Autodesk Inventor part; units mm, degrees
ref_plane "YZ Plane" through (0, 0, 0) normal (1, 0, 0) x (0, 1, 0)
ref_plane "XZ Plane" through (0, 0, 0) normal (0, 1, 0) x (-1, 0, 0)
ref_plane "XY Plane" through (0, 0, 0) normal (0, 0, 1) x (1, 0, 0)
sketch "Sketch1" plane through (0, 0, 0) normal (0, 0, 1) x (1, 0, 0)
  line L0 (17.9921, 17.8802) -> (17.9921, -20.5689)
  line L1 (-32.0079, 4.8802) -> (-32.0079, 14.8802) construction
  line L2 (-32.0079, 14.8802) -> (-22.0079, 14.8802) construction
  line L3 (-22.0079, 14.8802) -> (-22.0079, 4.8802) construction
  line L4 (-22.0079, 4.8802) -> (-32.0079, 4.8802) construction
  line L5 (-32.0079, 4.8802) -> (-32.0079, 14.8802) construction
  line L6 (17.9921, 14.8802) -> (-31.6168, 14.8802) construction
  line L7 (-31.6168, 4.8802) -> (18.3832, 4.8802) construction
  line L8 (-22.0079, 14.8802) -> (17.9921, 14.8802)
  line L9 (17.9921, 11.8802) -> (-22.0079, 11.8802)
  line L10 (-22.0079, 11.8802) -> (-22.0079, 14.8802)
  line L11 (17.9921, 14.8802) -> (17.9921, 11.8802)
  line L12 (-25.0079, 14.8802) -> (17.9921, 14.8802)
  line L13 (17.9921, 14.8802) -> (17.9921, 17.8802)
  line L14 (17.9921, 17.8802) -> (-25.0079, 17.8802)
  line L15 (-25.0079, 17.8802) -> (-25.0079, 14.8802)
  point P0 (0, 0)
  dimension "d2" = 10
  dimension "d13" = 10
  dimension "d52" = 3
  dimension "d53" = 0
  dimension "d55" = 80
  dimension "d56" = 40
  dimension "d57" = 3
  dimension "d58" = 3
revolve "Revolution1" add sketch "Sketch1" angle 360 about axis through (17.9921, 17.8802, 0) along (0, -1, 0)
sketch "Sketch3" plane through (17.9921, 11.8802, 0) normal (0, -1, 0) x (1, 0, 0)
  circle A0 centre (0, 0) radius 40
  line L0 (0, 40) -> (0, -38.6275)
  line L1 (-39.9999, 0.0946) -> (39.9999, 0.0946)
  circle A1 centre (10, 0.0946) radius 2
  circle A2 centre (20, 0.0946) radius 2
  circle A3 centre (30, 0.0946) radius 2
  circle A4 centre (4.9181, 8.7075) radius 2
  circle A5 centre (9.9181, 17.3678) radius 2
  circle A6 centre (14.9181, 26.028) radius 2
  circle A7 centre (-5.0819, 8.613) radius 2
  circle A8 centre (-10.0819, 17.2732) radius 2
  circle A9 centre (-15.0819, 25.9335) radius 2
  circle A10 centre (-10, -0.0946) radius 2
  circle A11 centre (-20, -0.0946) radius 2
  circle A12 centre (-30, -0.0946) radius 2
  circle A13 centre (-4.9181, -8.7075) radius 2
  circle A14 centre (-9.9181, -17.3678) radius 2
  circle A15 centre (-14.9181, -26.028) radius 2
  circle A16 centre (5.0819, -8.613) radius 2
  circle A17 centre (10.0819, -17.2732) radius 2
  circle A18 centre (15.0819, -25.9335) radius 2
  circle A19 centre (0, 35.25) radius 1.75
  circle A20 centre (-30.5274, -17.625) radius 1.75
  circle A21 centre (30.5274, -17.625) radius 1.75
  circle A22 centre (0, 0) radius 37 construction
  point P0 (-17.9921, 0)
  dimension "d59" = 4
  dimension "d60" = 10
  dimension "d66" = 10
  dimension "d70" = 360
  dimension "d72" = 3.5
  dimension "d75" = 360
  dimension "d80" = 3
extrude "Extrusion2" cut sketch "Sketch3" against normal through all contours A3 L1 | L1 A3 | A12 L1 | L1 A12 | A19 L0 | L0 A19 | A2 L1 | L1 A2 | A11 L1 | L1 A11 | A10 L1 | L1 A10 | A1 L1 | L1 A1 | A4 | A5 | A6 | A7 | A8 | A9 | A13 | A14 | A15 | A16 | A17 | A18 | A20 | A21
properties part number "bearing-base-uppercase"
Can you work these out from the model? Positions are in its coordinate system, mm. Round coordinates to 2 decimals unless told otherwise and drop trailing zeros. Order: outer loops, then holes, each group sorted by start corner. A loop starts at its lowest first (then second) coordinate and runs counter-clockwise, first axis right, second up. Notation, with made-up numbers: (-12.75, -32) -> (-7.75, -32) arc R23 ccw to (-7.75, -1) -> close; hole circle Ø7 at (-37, 75). An arc over 180 degrees is marked (long way). Return JSON: item names as keys, results as strings. Group by question number.
1. If we section it at D-D, the plane x = -8.5: Write out the boundary of the cut face in (y, z), then the cut area to 3 significant figures.
2. Will these pins go through, and if not, where does the flat tip stop? pin 1 (3 mm diameter, centred on x = 12.91, z = 8.61, fed in from +Y); pin 2 (2 mm diameter, centred on y = 13.5, z = -12.5, fed in from -X); pin 3 (1 mm diameter, centred on x = 27, y = 16.5, fed in from -Z).
3. If we section it at B-B, the plane x = 2.5: Write out the boundary of the cut face in (y, z).
4. If we section it at C-C, the plane z = -30: Write out the boundary of the cut face in (x, y), then the cut area to 3 significant figures.
5. I need wall thicknesses on line 1 (Z direction, x = 9, y = 12.8); line 2 (Z direction, x = 29.5, y = 13.6); line 3 (X direction, y = 16.5, z = 20). Which ranges of each line are inside material? Lowest first, please. Write a range as [from, to].
6. We'd pull the mould along Z, two halves only. Please class faces 1 (the face through (31.487, 14.838, -27.15)), 2 (the face through (57.953, 13.401, 1.759)), 3 (the face through (-20, 14.88, 13)), 4 (the face through (-12.76, 14.84, -15.89)): released by +Z, released by -Z, zero draft, split by the parting line, or undercut.
7. If we section it at A-A, the plane z = 35.25: Write out the boundary of the cut face in (x, y), then the cut area to 3 significant figures.
Output values:
{
 "1": {"outline": "(11.88, -29.97) -> (14.88, -29.97) -> (14.88, -33.87) -> (17.88, -33.87) -> (17.88, 33.87) -> (14.88, 33.87) -> (14.88, 29.97) -> (11.88, 29.97) -> close", "area": "383 mm²"},
 "2": {"pin 1": "through", "pin 2": "x = -20.32", "pin 3": "z = -42.15"},
 "3": {"outline": "(11.88, -36.88) -> (14.88, -36.88) -> (14.88, -40.11) -> (17.88, -40.11) -> (17.88, -27.94) -> (11.88, -27.94) -> close; (11.88, -24.11) -> (17.88, -24.11) -> (17.88, 23.98) -> (11.88, 23.98) -> close; (11.88, 27.89) -> (17.88, 27.89) -> (17.88, 40.11) -> (14.88, 40.11) -> (14.88, 36.88) -> (11.88, 36.88) -> close"},
 "4": {"outline": "(-12.81, 14.88) -> (-8.47, 14.88) -> (-8.47, 11.88) -> (44.45, 11.88) -> (44.45, 14.88) -> (48.8, 14.88) -> (48.8, 17.88) -> (-12.81, 17.88) -> close", "area": "344 mm²"},
 "5": {"line 1": "[-38.98, -19.14], [-15.6, -1.82], [1.63, 15.6], [18.95, 38.98]", "line 2": "[-38.31, -18.68], [-15.87, -1.22], [1.41, 16.15], [18.58, 38.31]", "line 3": "[-20.07, 56.06]"},
 "6": {"face 1": "undercut", "face 2": "split by the parting line", "face 3": "zero draft", "face 4": "undercut"},
 "7": {"outline": "(-6.63, 14.88) -> (-0.91, 14.88) -> (-0.91, 11.88) -> (16.24, 11.88) -> (16.24, 17.88) -> (-6.63, 17.88) -> close; (19.74, 11.88) -> (36.9, 11.88) -> (36.9, 14.88) -> (42.62, 14.88) -> (42.62, 17.88) -> (19.74, 17.88) -> close", "area": "240 mm²"}
}
